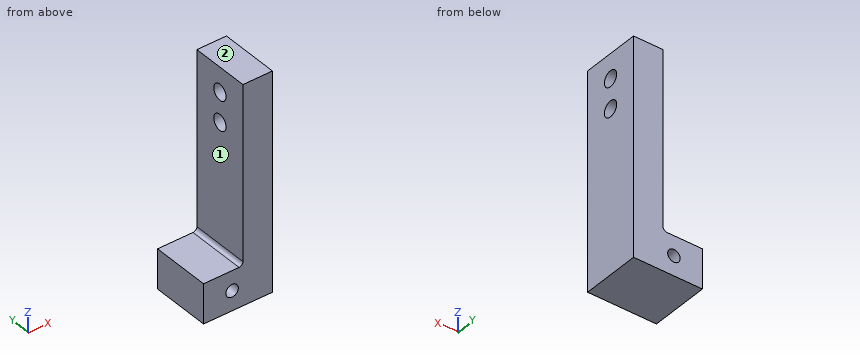
Autodesk Inventor part; units mm, degrees
ref_plane "YZ Plane" through (0, 0, 0) normal (1, 0, 0) x (0, 1, 0)
ref_plane "XZ Plane" through (0, 0, 0) normal (0, 1, 0) x (-1, 0, 0)
ref_plane "XY Plane" through (0, 0, 0) normal (0, 0, 1) x (1, 0, 0)
sketch "Sketch1" plane through (0, 0, 0) normal (0, 0, 1) x (1, 0, 0)
  line L0 (0, 0) -> (35, 0)
  line L1 (35, 0) -> (35, 30)
  line L2 (35, 30) -> (0, 30)
  line L3 (0, 30) -> (0, 0)
  dimension "d0" = 35
  dimension "d1" = 30
extrude "Extrusion1" add sketch "Sketch1" along normal blind 110
sketch "Sketch2" plane through (0, 0, 110) normal (0, 0, 1) x (1, 0, 0)
  line L0 (0, 0) -> (35, 0)
  line L1 (35, 0) -> (35, 30)
  line L2 (35, 30) -> (0, 30)
  line L3 (0, 30) -> (0, 0)
  line L4 (0, 0) -> (35, 0)
  line L5 (35, 30) -> (20, 30)
  line L6 (20, 30) -> (20, 0)
  line L7 (20, 0) -> (35, 0)
  line L8 (35, 0) -> (35, 30)
  dimension "d4" = 15
extrude "Extrusion2" cut sketch "Sketch2" against normal blind 90 contours L3 L2 L6 L0
sketch "Sketch3" plane through (35, 0, 0) normal (1, 0, 0) x (0, 0, -1)
  line L0 (0, 0) -> (0, 30)
  line L1 (0, 30) -> (-110, 30)
  line L2 (-110, 0) -> (-110, 30)
  line L3 (0, 0) -> (-110, 0)
  circle A0 centre (-97.5, 15) radius 4
  circle A1 centre (-82.5, 15) radius 4
  point P0 (0, 0)
  dimension "d9" = 15
  dimension "d10" = 15
  dimension "d11" = 12.5
  dimension "d12" = 15
  dimension "d13" = 8
  dimension "d14" = 8
extrude "Extrusion3" cut sketch "Sketch3" against normal up to next contours A0 | A1
sketch "Sketch4" plane through (0, 30, 0) normal (0, 1, 0) x (1, 0, 0)
  circle A0 centre (14.5, -10) radius 3.175
  line L0 (0, 0) -> (0, -20)
  line L1 (0, -20) -> (20, -20)
  line L2 (35, 0) -> (0, 0)
  dimension "d17" = 6.35
  dimension "d18" = 14.5
  dimension "d23" = 10
extrude "Extrusion4" cut sketch "Sketch4" against normal up to next
fillet "Fillet1" radius 2 1 edges at (20, 15, 20)
properties part number "X_Rail_Belt_Pulley_Connector"
Work out the finished part from the listing and answer in its coordinate system (mm). Face numbers are marked on the shaded views. A direction names the side the tool comes from. Give positions to 0.01 mm unless a question says otherwise; leave off trailing zeros. Order: outer loops, then holes, each group sorted by start corner. A loop starts at its lowest first (then second) coordinate and runs counter-clockwise, first axis right, second up. Notation, with made-up numbers: (34.25, -12) -> (76.25, -12) arc R30 ccw to (76.25, 22) -> close; hole circle Ø2 at (30, 15). An arc over 180 degrees is marked (long way). Answer as CSV lines item,"result". Start each with the question number.
(1) Section B-B, the plane z = 10 is taken. Write down the section's boundary in (x, y) (3 decimals), plus the area to 4 significant figures.
(2) Section A-A, the plane y = 15 is taken. Write down the section's boundary in (x, z) (3 decimals).
(3) Each of these flat-tipped pins is pushed along its axis until it touches: pin 1 Ø10 at (y, z) = (26.5, 28.5) entering from -X; pin 2 Ø5 at (y, z) = (15, 82.5) entering from -X. Where does it stop, or does it pass through?
(4) Which of the six approach directions +Z, -Z, +X, -X, +Y, -Y give full straight-line access (tool end or side, diameter ignored) to the marked faces 1 and 2?
(5) Section C-C, the plane x = 14.5 is taken. Write down the section's boundary in (y, z) (3 decimals), plus the area to 4 significant figures.
(6) Section D-D, the plane y = 21.75 is taken. Write down the section's boundary in (x, z) (3 decimals).
(7) Consider line 1 along Z through (x, y) = (33.5, 15.25); line 2 along X through (y, z) = (13.25, 10) (3 decimals); line 3 along Z through (x, y) = (23.5, 11.75). Determine where each line is inside the solid, lowest interval first.
Entries:
1,outline,"(0, 0) -> (11.325, 0) -> (11.325, 30) -> (0, 30) -> close; (17.675, 0) -> (35, 0) -> (35, 30) -> (17.675, 30) -> close"
1,area,"859.5 mm²"
2,outline,"(0, 0) -> (35, 0) -> (35, 78.5) -> (20, 78.5) -> (20, 22) arc R2 cw to (18, 20) -> (0, 20) -> close; (20, 86.5) -> (35, 86.5) -> (35, 93.5) -> (20, 93.5) -> close; (20, 101.5) -> (35, 101.5) -> (35, 110) -> (20, 110) -> close; hole circle Ø6.35 at (14.5, 10)"
3,pin 1,"x = 20"
3,pin 2,"through"
4,face 1,"+Z, -X, +Y, -Y"
4,face 2,"+Z, +X, -X, +Y, -Y"
5,outline,"(0, 0) -> (30, 0) -> (30, 6.825) -> (0, 6.825) -> close; (0, 13.175) -> (30, 13.175) -> (30, 20) -> (0, 20) -> close"
5,area,"409.5 mm²"
6,outline,"(0, 0) -> (35, 0) -> (35, 110) -> (20, 110) -> (20, 22) arc R2 cw to (18, 20) -> (0, 20) -> close; hole circle Ø6.35 at (14.5, 10)"
7,line 1,"0 to 78.51, 86.49 to 93.51, 101.49 to 110"
7,line 2,"0 to 11.325, 17.675 to 35"
7,line 3,"0 to 80.17, 84.83 to 95.17, 99.83 to 110"
